Geometry: final body of the model. Coordinates: model frame, mm. A direction names the side the tool comes from. Round coordinates to 2 decimals unless told otherwise and drop trailing zeros. Loops run counter-clockwise (first coordinate to the right, second up) from the corner with the lowest first, then second, coordinate; pieces in that order, holes last. Notation, with made-up numbers: (84, 15.25) -> (113, 15.25) arc R22 ccw to (113, 35.25) -> close; hole circle Ø5 at (33, -6.75). An arc over 180 degrees is marked (long way). Answer in a Markdown table with one row per item.
```python
from build123d import *

# Parameters (mm, degrees)
ESBO_O1_R                  = 1.6
RESSALTO_EXTRUS_O1_DEPTH   = 50
ESBO_O2_W                  = 20
ESBO_O2_H                  = 20
CORTE_EXTRUS_O1_DEPTH      = 43
ESBO_O3_R                  = 1.65
CORTE_EXTRUS_O2_DEPTH      = 22
CORTE_EXTRUS_O2_DEPTH_BACK = 27
ESBO_O6_R                  = 1.65
CORTE_EXTRUS_O4_DEPTH      = 18.2
FILETE1_R                  = 2
ESBO_O4_R                  = 6.5
CORTE_EXTRUS_O5_DEPTH      = 24
CORTE_EXTRUS_O6_DEPTH      = 1
ESBO_O8_R                  = 5.25
CORTE_EXTRUS_O7_DEPTH      = 1
ESBO_O9_R                  = 5.25
CORTE_EXTRUS_O8_DEPTH      = 1


with BuildPart() as part:
    # Esboço1 → Ressalto-extrusão1 (new body)
    with BuildSketch(Plane.XY):
        with BuildLine():
            Line((0, 0), (0, 11))
            Line((0, 11), (-26, 11))
            Line((-26, 11), (-26, 0))
            Line((-26, 0), (-35, 0))
            ThreePointArc((-35, 0), (-46.699949915, -9.333321918), (-40.2, -22.814804668))
            Line((-40.2, -22.814804668), (-40.2, -31))
            Line((-40.2, -31), (-35.7, -31))
            Line((-35.7, -31), (-35.7, -19.567694497))
            ThreePointArc((-35.7, -19.567694497), (-35, -4.4), (-34.3, -19.567694497))
            Line((-34.3, -19.567694497), (-34.3, -31))
            Line((-34.3, -31), (-29.8, -31))
            Line((-29.8, -31), (-29.8, -24))
            Line((-29.8, -24), (0, -24))
            Line((0, -24), (0, 0))
        make_face()
        with Locations((-10, -6.5)):
            Circle(ESBO_O1_R, mode=Mode.SUBTRACT)
    extrude(amount=RESSALTO_EXTRUS_O1_DEPTH)

    # Esboço2 → Corte-extrusão1 (cut, through all)
    with BuildSketch(Plane(origin=(0, 11, 0), x_dir=(1, 0, 0), z_dir=(0, 1, 0))):
        Polygon((0, -24), (-20, -50), (0, -50), align=None)
        with Locations((-10, -10)):
            Rectangle(ESBO_O2_W, ESBO_O2_H)
    extrude(amount=-CORTE_EXTRUS_O1_DEPTH, mode=Mode.SUBTRACT)

    # Esboço3 → Corte-extrusão2 (cut, two sides)
    with BuildSketch(Plane.ZY.offset(26)) as corte_extrus_o2_sk:
        with Locations((10, 5.5)):
            Circle(ESBO_O3_R)
        Polygon((50, -24), (43, -31), (50, -31), align=None)
        Polygon((50, 0), (24, 11), (50, 11), align=None)
        Polygon((0, -24), (0, -31), (7, -31), align=None)
        Polygon((7, 11), (0, 4), (0, 11), align=None)
    extrude(amount=CORTE_EXTRUS_O2_DEPTH, mode=Mode.SUBTRACT)
    extrude(corte_extrus_o2_sk.sketch, amount=-CORTE_EXTRUS_O2_DEPTH_BACK, mode=Mode.SUBTRACT)

    # Esboço6 → Corte-extrusão4 (cut, through all)
    with BuildSketch(Plane(origin=(-29.8, 0, 0), x_dir=(0, 0, -1), z_dir=(1, 0, 0))):
        with Locations((-38, -27.5)):
            Circle(ESBO_O6_R)
        with Locations((-12, -27.5)):
            Circle(ESBO_O6_R)
    extrude(amount=-CORTE_EXTRUS_O4_DEPTH, mode=Mode.SUBTRACT)

    # Filete1
    filete1_edges = [part.edges().sort_by_distance(p)[0] for p in [
        (-34.3, -19.567694497, 25),
        (-35.7, -19.567694497, 25),
    ]]
    fillet(filete1_edges, radius=FILETE1_R)

    # Esboço4 → Corte-extrusão5 (cut)
    with BuildSketch(Plane.XY.offset(50)):
        with Locations((-10, -6.5)):
            Circle(ESBO_O4_R)
    extrude(amount=-CORTE_EXTRUS_O5_DEPTH, mode=Mode.SUBTRACT)

    # Esboço7 → Corte-extrusão6 (cut)
    with BuildSketch(Plane(origin=(-29.8, 0, 0), x_dir=(0, 0, -1), z_dir=(1, 0, 0))):
        Polygon((-8.824573519, -27.5), (-10.41228676, -24.75), (-13.58771324, -24.75), (-15.175426481, -27.5), (-13.58771324, -30.25), (-10.41228676, -30.25), align=None)
        Polygon((-34.824573519, -27.5), (-36.41228676, -24.75), (-39.58771324, -24.75), (-41.175426481, -27.5), (-39.58771324, -30.25), (-36.41228676, -30.25), align=None)
    extrude(amount=-CORTE_EXTRUS_O6_DEPTH, mode=Mode.SUBTRACT)

    # Esboço8 → Corte-extrusão7 (cut)
    with BuildSketch(Plane(origin=(-20, 0, 0), x_dir=(0, 0, -1), z_dir=(1, 0, 0))):
        with Locations((-10, 5.5)):
            Circle(ESBO_O8_R)
    extrude(amount=-CORTE_EXTRUS_O7_DEPTH, mode=Mode.SUBTRACT)

    # Esboço9 → Corte-extrusão8 (cut)
    with BuildSketch(Plane(origin=(0, 0, 20), x_dir=(-1, 0, 0), z_dir=(0, 0, -1))):
        with Locations((10, -6.5)):
            Circle(ESBO_O9_R)
    extrude(amount=-CORTE_EXTRUS_O8_DEPTH, mode=Mode.SUBTRACT)


solid = part.part
```
Item 1: Line query: probe 1 along X at (y, z) = (-27, 16.5); probe 2 along Y at (x, z) = (-20.45, 10); probe 3 along Y at (x, z) = (-38.85, 38). Output: solid intervals per line, ascending. Write a range as [from, to].
Answer:
| item | result |
|---|---|
| probe 1 | x = [-40.2, -35.7], [-34.3, -29.8] |
| probe 2 | y = [-24, 0.25], [10.75, 11] |
| probe 3 | y = [-31, -29.15], [-25.85, -18.55], [-5.45, -0.63] |
Item 2: Cut plane C-C (z = 23). Output: boundary loops of the cut face in (x, y), then the cut area to 3 significant figures.
Answer:
| item | result |
|---|---|
| outline | (-40.2, -31) -> (-35.7, -31) -> (-35.7, -21.21) arc R2 ccw to (-37.14, -19.29) arc R7.6 cw (long way) to (-32.86, -19.29) arc R2 ccw to (-34.3, -21.21) -> (-34.3, -31) -> (-29.8, -31) -> (-29.8, -24) -> (0, -24) -> (0, 11) -> (-26, 11) -> (-26, 0) -> (-35, 0) arc R12 ccw to (-40.2, -22.81) -> close; hole circle Ø3.2 at (-10, -6.5) |
| area | 1,220 mm² |
Item 3: Reachability of faces 1 (the face through (-33.89, -20, 25.35)), 2 (the face through (-35.7, -26, 25)), 3 (the face through (-30.29, -28.86, 14.39)) from +Z, -Z, +X, -X, +Y, -Y: full face, straight path, thin tool, end or side. Return the list, or none.
Answer:
| item | result |
|---|---|
| face 1 | +Z, -Z |
| face 2 | +Z, -Z, -Y |
| face 3 | +X |
Item 4: Cut plane B-B (z = 38). Count the separate pieces of the cut face and the enclosed holes in it, then the cut area to 3 significant figures.
Answer:
| item | result |
|---|---|
| separate pieces | 3 |
| enclosed holes | 0 |
| area | 673 mm² |
Item 5: Draft query along X for faces 4 (the face through (-30.29, -26.14, 35.61)), 5 (the face through (0, -7, 22)), 6 (the face through (-9, -8, 26)). Return one class per face: pulls with the +X half, pulls with the -X half, needs draft (parallel to the pull), parting line crosses it, or undercut.
Answer:
| item | result |
|---|---|
| face 4 | needs draft |
| face 5 | pulls with the +X half |
| face 6 | undercut |
Item 6: Cut plane D-D (y = -16). Output: boundary loops of the cut face in (x, z).
Answer:
| item | result |
|---|---|
| outline | (-46.31, 0) -> (-41.46, 0) -> (-41.46, 50) -> (-46.31, 50) -> close; (-28.54, 0) -> (-20, 0) -> (-20, 20) -> (0, 20) -> (0, 24) -> (-20, 50) -> (-28.54, 50) -> close |
Item 7: Pin query (flat end, axial travel): pin 1 Ø7 at (x, z) = (-32.5, 23.5) entering from +Y; pin 2 Ø6 at (x, y) = (-9, -14.5) entering from -Z; pin 3 Ø12 at (x, y) = (-4.5, -15.5) entering from +Z; pin 4 Ø5 at (x, z) = (-28, 42) entering from -Y. Return the tip coordinate at first contact, or that it passes through.
Answer:
| item | result |
|---|---|
| pin 1 | stops at y = 0 |
| pin 2 | stops at z = 20 |
| pin 3 | stops at z = 37.65 |
| pin 4 | stops at y = -31 |
Item 8: Cut plane A-A (x = -10). Output: boundary loops of the cut face in (y, z).
Answer:
| item | result |
|---|---|
| outline | (-24, 20) -> (-11.75, 20) -> (-11.75, 21) -> (-8.1, 21) -> (-8.1, 26) -> (-13, 26) -> (-13, 37) -> (-24, 37) -> close; (-4.9, 21) -> (-1.25, 21) -> (-1.25, 20) -> (11, 20) -> (11, 24) -> (5.5, 37) -> (0, 37) -> (0, 26) -> (-4.9, 26) -> close |
